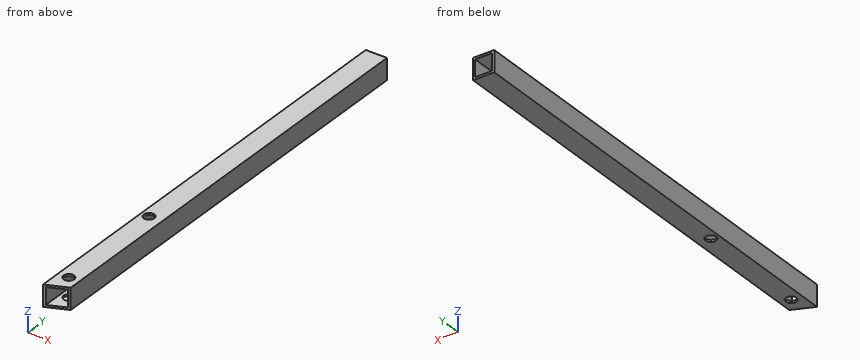
Autodesk Inventor part; units mm, degrees
ref_plane "YZ Plane" through (0, 0, 0) normal (1, 0, 0) x (0, 1, 0)
ref_plane "XZ Plane" through (0, 0, 0) normal (0, 1, 0) x (-1, 0, 0)
ref_plane "XY Plane" through (0, 0, 0) normal (0, 0, 1) x (1, 0, 0)
sketch "Sketch1" plane through (0, 0, 0) normal (0, 1, 0) x (-1, 0, 0)
  line L0 (12.7, 12.7) -> (-12.7, 12.7)
  line L1 (-12.7, 12.7) -> (-12.7, -12.7)
  line L2 (-12.7, -12.7) -> (12.7, -12.7)
  line L3 (12.7, -12.7) -> (12.7, 12.7)
  line L4 (12.7, 12.7) -> (-12.7, -12.7) construction
  line L5 (-12.7, 12.7) -> (12.7, -12.7) construction
  line L6 (10.16, 10.16) -> (-10.16, 10.16)
  line L7 (-10.16, 10.16) -> (-10.16, -10.16)
  line L8 (-10.16, -10.16) -> (10.16, -10.16)
  line L9 (10.16, -10.16) -> (10.16, 10.16)
  point P0 (0, 0)
  dimension "d0" = 25.4
  dimension "d1" = 25.4
  dimension "d2" = 2.54
extrude "Extrusion1" add sketch "Sketch1" along normal blind 635
sketch "Sketch2" plane through (-12.7, 0, 12.7) normal (0, 0, 1) x (1, 0, 0)
  line L0 (-200.1642, 538.812) -> (-221.8597, 525.6033) construction
  line L1 (-221.8597, 525.6033) -> (42.3138, 91.695) construction
  line L2 (64.0092, 104.9037) -> (42.3138, 91.695) construction
  line L3 (-200.1642, 538.812) -> (64.0092, 104.9037) construction
  line L4 (0, 0) -> (25.4, 0) construction
  line L5 (25.4, 0) -> (25.4, 635)
  line L6 (0, 635) -> (25.4, 635) construction
  line L7 (0, 0) -> (0, 635) construction
  line L8 (-200.1642, 538.812) -> (-221.8597, 525.6033) construction
  line L9 (-221.8597, 525.6033) -> (42.3138, 91.695) construction
  line L10 (64.0092, 104.9037) -> (42.3138, 91.695) construction
  line L11 (-200.1642, 538.812) -> (64.0092, 104.9037) construction
  line L12 (25.4, 0) -> (25.4, 635) construction
  line L13 (0, 0) -> (0, 635) construction
  line L14 (0, 95.9598) -> (0, 0) construction
  line L15 (0, 0) -> (25.4, 0) construction
  line L16 (25.4, 0) -> (25.4, 106.7696) construction
  line L17 (22.86, 0) -> (22.86, 635) construction
  line L18 (25.4, 0) -> (25.4, 635) construction
  line L19 (25.4073, 106.776) -> (0, 95.9598)
  line L20 (0, 0) -> (0, 95.9598)
  line L21 (2.54, 0) -> (2.54, 635)
  line L22 (0, 0) -> (25.4, 0)
  line L23 (25.4, 0) -> (25.4073, 106.776)
  line L24 (25.4, 0) -> (25.4073, 0.0057)
  line L25 (25.4073, 0.0057) -> (25.4073, 106.776)
  circle A0 centre (46.5571, 109.1471) radius 6.35
  circle A1 centre (46.5571, 109.1471) radius 6.35
  point P0 (12.7, 0)
extrude "Extrusion2" cut sketch "Sketch2" against normal blind 128.5875 contours L22 L21 L19 L5 | L5 L19 L23 | L23 L25 L24 | L22 L20 L19 L21
sketch "Sketch4" plane through (-12.7, 635, 12.7) normal (0, 0, 1) x (1, 0, 0)
  circle A0 centre (46.5571, -525.8529) radius 6.35
  point P0 (12.7, -635)
extrude "Extrusion3" cut sketch "Sketch4" against normal blind 128.5875
sketch "Sketch5" plane through (-12.7, 635, 12.7) normal (0, 0, 1) x (1, 0, 0)
  circle A0 centre (9.7002, -375.3859) radius 6.35
  point P0 (12.7, -635)
extrude "Extrusion4" cut sketch "Sketch5" against normal through all
sketch "Sketch6" plane through (-12.7, 635, 12.7) normal (0, 0, 1) x (1, 0, 0)
  circle A0 centre (12.7, -513.6388) radius 6.35
  point P0 (12.7, -635)
  dimension "d11" = 12.7
extrude "Extrusion5" cut sketch "Sketch6" against normal through all
equation "\"BendRadius\" = Thickness"
equation "\"BendReliefWidth\" = Thickness"
equation "\"BendReliefDepth\" = 0.5 * Thickness"
equation "\"CornerReliefSize\" = 4 * Thickness"
equation "\"MinimumRemnant\" = 2 * Thickness"
equation "\"TransitionRadius\" = BendRadius"
equation "\"JacobiRadiusSize\" = BendRadius"
equation "\"GapSize\" = Thickness"
properties part number "conveyer frame" material "Aluminum 6061"
CAD build for the part. Positions are in the model's coordinates, mm. Round coordinates to 2 decimals unless told otherwise and drop trailing zeros. Order: outer loops, then holes, each group sorted by start corner. A loop starts at its lowest first (then second) coordinate and runs counter-clockwise, first axis right, second up.
Q1. Wall check: L1, parallel to X at y = 210.5, z = -9.75; L2, parallel to Y at x = 0, z = 11.65. Give the ranges that are in metal, low to high.
Q2. Slice it at B-B (x = -2.25). Write the cut outline in (y, z), and give its area (3 significant figures).
Q3. Drop a flat-ended pin along its axis: pin 1 (2 mm diameter, centred on x = -9.5, z = -9.5, fed in from -Y). Give the stop position or say it passes through.
Q4. Slice it at A-A (y = 468). Write the cut outline in (x, z), and give its area (3 significant figures).
Results below:
1. L1: x = -12.7 to -10.16, 10.16 to 12.7
1. L2: y = 101.37 to 115.01, 127.71 to 254.02, 265.21 to 635
2. outline: (100.41, -12.7) - (115.42, -12.7) - (115.42, -10.16) - (100.41, -10.16) - close; (100.41, 10.16) - (115.42, 10.16) - (115.42, 12.7) - (100.41, 12.7) - close; (127.3, -12.7) - (253.31, -12.7) - (253.31, -10.16) - (127.3, -10.16) - close; (127.3, 10.16) - (253.31, 10.16) - (253.31, 12.7) - (127.3, 12.7) - close; (265.92, -12.7) - (635, -12.7) - (635, -10.16) - (265.92, -10.16) - close; (265.92, 10.16) - (635, 10.16) - (635, 12.7) - (265.92, 12.7) - close
2. area: 2,590 mm2
3. pin 1: stops at y = 96.9
4. outline: (-12.7, -12.7) - (12.7, -12.7) - (12.7, 12.7) - (-12.7, 12.7) - close; hole (-10.16, -10.16) - (10.16, -10.16) - (10.16, 10.16) - (-10.16, 10.16) - close
4. area: 232 mm2
